Input: part model. Units: mm. Frame: model coordinates. A direction names the side the tool comes from. Give positions to 0.01 mm unless a question says otherwise; leave off trailing zeros. Loops run counter-clockwise (first coordinate to the right, second up) from the corner with the lowest first, then second, coordinate; pieces in that order, holes last. Notation, with made-up numbers: (38, 56) - (82, 56) arc R22 ccw to (82, 67) - close; hole circle Ø10 at (-25.75, -24). An arc over 180 degrees is marked (long way). Answer as a JSON object with one key per item and string values. Group by question number.
(1) Pin query (flat end, axial travel): P1, Ø6, axis at x = 14, y = 20, coming from the -Z side. Return the tip coordinate at first contact, or that it passes through.
(2) Section query A-A (x = 25.4). Count the separate pieces of the cut face and the enclosed holes in it, plus the area to 3 significant figures.
(3) Access query for faces 4 (the flat face through (3.175, 13, 351)), 5 (the cylindrical face through (23.747, 1.61, 165.208)). Directions: +Z, -Z, +X, -X, +Y, -Y. A direction counts if a zero-diameter tool reaches every point of the face in a straight line with its end or side. Return the directions, or none.
(4) Section query C-C (y = 14.5). Return loops of the section in (x, z) (3 decimals).
(5) Section query B-B (z = 397). Return loops of the section in (x, y) (3 decimals).
(6) Section query D-D (z = 177.8). Return loops of the section in (x, y) (3 decimals), plus the area to 3 significant figures.
(7) Mould query, pull axis Y, two halves, no side actions, for faces 1 (the flat face through (42, 0, 351)), 2 (the flat face through (47.625, 13, 351)), 3 (the flat face through (50.8, 13, 351)). Classes: +Y half, -Y half, draft (parallel to the pull), parting line (faces both ways), or undercut.
(8) Material intervals for L1, parallel to Z at x = 25.4, y = 2.55; L2, parallel to X at y = 18.75, z = 399 (3 decimals); L3, parallel to X at y = 24.7, z = 355.6, sorted ascending.
Autodesk Inventor part; units mm, degrees
ref_plane "YZ Plane" through (0, 0, 0) normal (1, 0, 0) x (0, 1, 0)
ref_plane "XZ Plane" through (0, 0, 0) normal (0, 1, 0) x (-1, 0, 0)
ref_plane "XY Plane" through (0, 0, 0) normal (0, 0, 1) x (1, 0, 0)
sketch "Sketch1" plane through (0, 0, 0) normal (0, 0, 1) x (1, 0, 0)
  line L0 (0, 0) -> (50.8, 0)
  line L1 (50.8, 0) -> (50.8, 25.4)
  line L2 (50.8, 25.4) -> (0, 25.4)
  line L3 (0, 25.4) -> (0, 0)
  line L4 (3.175, 22.225) -> (47.625, 22.225)
  line L5 (47.625, 22.225) -> (47.625, 3.175)
  line L6 (47.625, 3.175) -> (3.175, 3.175)
  line L7 (3.175, 3.175) -> (3.175, 22.225)
  dimension "d0" = 50.8
  dimension "d1" = 25.4
  dimension "d2" = 3.175
extrude "Extrusion1" add sketch "Sketch1" along normal blind 711.2
sketch "Sketch2" plane through (0, 25.4, 0) normal (0, 1, 0) x (1, 0, 0)
  line L0 (0, 0) -> (0, -711.2)
  line L1 (0, -355.6) -> (50.8, -355.6)
  line L2 (50.8, 0) -> (50.8, -711.2)
  line L3 (50.8, -711.2) -> (0, -711.2)
  line L4 (0, -355.6) -> (0, -711.2)
  line L5 (0, -533.4) -> (50.8, -533.4)
  line L6 (0, -355.6) -> (0, 0)
  line L7 (0, -177.8) -> (50.8, -177.8)
  circle A0 centre (25.4, -533.4) radius 12.7
  circle A1 centre (25.4, -355.6) radius 12.7
  circle A2 centre (25.4, -177.8) radius 12.7
  dimension "d5" = 25.4
extrude "Extrusion2" cut sketch "Sketch2" against normal blind 25.4 contours A2 L7 | L7 A2 | A1 L1 | L1 A1 | A0 L5 | L5 A0
properties part number "1x2x28"
Recorded:
{
 "1": {"P1": "stops at z = 0"},
 "2": {"separate pieces": "8", "enclosed holes": "0", "area": "4,030 mm^2"},
 "3": {"face 4": "+Z, -Z", "face 5": "+Y, -Y"},
 "4": {"outline": "(0, 0) - (3.175, 0) - (3.175, 711.2) - (0, 711.2) - close; (47.625, 0) - (50.8, 0) - (50.8, 711.2) - (47.625, 711.2) - close"},
 "5": {"outline": "(0, 0) - (50.8, 0) - (50.8, 25.4) - (0, 25.4) - close; hole (3.175, 3.175) - (47.625, 3.175) - (47.625, 22.225) - (3.175, 22.225) - close"},
 "6": {"outline": "(0, 0) - (12.7, 0) - (12.7, 3.175) - (3.175, 3.175) - (3.175, 22.225) - (12.7, 22.225) - (12.7, 25.4) - (0, 25.4) - close; (38.1, 0) - (50.8, 0) - (50.8, 25.4) - (38.1, 25.4) - (38.1, 22.225) - (47.625, 22.225) - (47.625, 3.175) - (38.1, 3.175) - close", "area": "282 mm^2"},
 "7": {"face 1": "-Y half", "face 2": "undercut", "face 3": "draft"},
 "8": {"L1": "z = 0 to 165.1, 190.5 to 342.9, 368.3 to 520.7, 546.1 to 711.2", "L2": "x = 0 to 3.175, 47.625 to 50.8", "L3": "x = 0 to 12.7, 38.1 to 50.8"}
}
